Autodesk Inventor part; units mm, degrees
ref_plane "YZ Plane" through (0, 0, 0) normal (1, 0, 0) x (0, 1, 0)
ref_plane "XZ Plane" through (0, 0, 0) normal (0, 1, 0) x (-1, 0, 0)
ref_plane "XY Plane" through (0, 0, 0) normal (0, 0, 1) x (1, 0, 0)
sketch "Skizze1" plane through (0, 0, 0) normal (0, 0, 1) x (1, 0, 0)
  line L0 (-19, -14.5) -> (-19, -10.5)
  line L1 (-19, -10.5) -> (-16.2321, -10.5)
  line L2 (-16.2321, -10.5) -> (-14.5, -7.5)
  line L3 (-14.5, -7.5) -> (-14.5, 0)
  line L4 (-14.5, 0) -> (14.5, 0)
  line L5 (14.5, 0) -> (14.5, -7.5)
  line L6 (14.5, -7.5) -> (16.2321, -10.5)
  line L7 (16.2321, -10.5) -> (22.5, -10.5)
  line L8 (22.5, -10.5) -> (22.5, -14.5)
  line L9 (22.5, -14.5) -> (28.5, -20.5)
  line L10 (28.5, -20.5) -> (32.5, -20.5)
  line L11 (32.5, -20.5) -> (32.5, 16.5)
  line L12 (32.5, 16.5) -> (-29, 16.5)
  line L13 (-29, 16.5) -> (-29, -20.5)
  line L14 (-29, -20.5) -> (-25, -20.5)
  line L15 (-25, -20.5) -> (-19, -14.5)
  line L16 (0, 0) -> (0, -29.3821)
  dimension "d5" = 29
  dimension "d6" = 16.5
  dimension "d7" = 7.5
  dimension "d8" = 4.5
  dimension "d10" = 41.5
  dimension "d12" = 30
  dimension "d13" = 10
  dimension "d14" = 10
  dimension "d15" = 10.5
  dimension "d16" = 45
  dimension "d17" = 10
  dimension "d18" = 4
extrude "Extrusion1" add sketch "Skizze1" along normal mid plane 10
chamfer "Fase1" distance 1 angle 45 2 edges at (-19, -12.5, -5) (-22, -17.5, -5)
properties part number "_WT_Aufnahme_Antriebseinheit4"
Here's how the part is built. I have some questions about the finished solid (model axes, mm). A direction names the side the tool comes from. Coordinates: 2 decimals unless noted, no trailing zeros. Order: outer loops, then holes, each group sorted by start corner. A loop starts at its lowest first (then second) coordinate and runs counter-clockwise, first axis right, second up. Notation, with made-up numbers: (3, 75) - (55, 75) arc R14 cw to (55, 87) - close; hole circle Ø11 at (83, 66). An arc over 180 degrees is marked (long way). One line per question, with ' | ' between items. Start each with the question number.
1. If we section it at A-A (y = -1): Write out the boundary of the cut face in (x, z), and give its area (3 significant figures).
2. Please list where these lines run through material, in increasing order: line 1 along X through (y, z) = (-0.5, -1); line 2 along Y through (x, z) = (17, 1.25); line 3 along Y through (x, z) = (10, -1.25). Write a range as [from, to].
3. Which directions (+Z, -Z, +X, -X, +Y, -Y) give clear straight access to the entire face, cutting with the end or side of a thin tool? Please do faces 5 (the flat face through (-14.5, -4, 0)), 6 (the flat face through (2, 16.5, 0)), 7 (the flat face through (-22.67, -17.45, -4.51)).
4. If we section it at B-B (z = 4.25): Write out the boundary of the cut face in (x, y).
5. If we mould it in two halves opening along X, with no side actions, what happens to faces 1 (the flat face through (32.5, -2, 0)), 2 (the flat face through (19, -10.5, 0)), 3 (the flat face through (25, -17, 0)), 4 (the flat face through (30, -20.5, 0))? For each: released by +X, released by -X, zero draft, split by the parting line, or undercut.
6. If we section it at D-D (y = -9.5): Write out the boundary of the cut face in (x, z).
7. I'm going to push flat-ended pins straight in: pin 1 Ø5 at (x, z) = (20.5, 0) entering from -Y; pin 2 Ø1.5 at (x, z) = (-6.5, -2) entering from -Y. Where does each tip first touch, or does it pass through?
8. If we section it at C-C (x = -9): Write out the boundary of the cut face in (y, z).
Model answer:
1) outline: (-29, -5) - (-14.5, -5) - (-14.5, 5) - (-29, 5) - close; (14.5, -5) - (32.5, -5) - (32.5, 5) - (14.5, 5) - close | area: 325 mm²
2) line 1: x = [-29, -14.5], [14.5, 32.5] | line 2: y = [-10.5, 16.5] | line 3: y = [0, 16.5]
3) face 5: +Z, -Z, -Y | face 6: +Z, -Z, +X, -X, +Y | face 7: -Z, -Y
4) outline: (-29, -20.5) - (-25, -20.5) - (-19, -14.5) - (-19, -10.5) - (-16.23, -10.5) - (-14.5, -7.5) - (-14.5, 0) - (14.5, 0) - (14.5, -7.5) - (16.23, -10.5) - (22.5, -10.5) - (22.5, -14.5) - (28.5, -20.5) - (32.5, -20.5) - (32.5, 16.5) - (-29, 16.5) - close
5) face 1: released by +X | face 2: undercut | face 3: undercut | face 4: zero draft
6) outline: (-29, -5) - (-15.65, -5) - (-15.65, 5) - (-29, 5) - close; (15.65, -5) - (32.5, -5) - (32.5, 5) - (15.65, 5) - close
7) pin 1: stops at y = -15 | pin 2: stops at y = 0
8) outline: (0, -5) - (16.5, -5) - (16.5, 5) - (0, 5) - close
